```python
from build123d import *

# Parameters (mm, degrees)
SKETCH_1_R          = 14
SKETCH_1_R_2        = 1.5
EXTRUDE_1_DEPTH     = 2
CUT_EXTRUDE_1_DEPTH = 20.899748742
EXTRUDE_4_DEPTH     = 1
SKETCH_6_R          = 7
SKETCH_6_R_2        = 3.1
EXTRUDE_5_DEPTH     = 5
EXTRUDE_6_DEPTH     = 1
SKETCH_8_W          = 8
SKETCH_8_H          = 2
EXTRUDE_7_DEPTH     = 5
SKETCH_9_R          = 1.6
CUT_EXTRUDE_3_DEPTH = 24.108440017
EXTRUDE_8_DEPTH     = 2
SKETCH_11_W         = 12.041493288
SKETCH_11_H         = 2
CUT_EXTRUDE_4_DEPTH = 5
SKETCH_12_R         = 20
SKETCH_12_R_2       = 3.1
EXTRUDE_9_DEPTH     = 2
SKETCH_13_R         = 2.3
CUT_EXTRUDE_5_DEPTH = 2
CUT_EXTRUDE_START   = -1
CUT_EXTRUDE_6_DEPTH = 1
FILLET_1_R          = 3
FILLET_2_R          = 1.5
SKETCH_15_R         = 20
CUT_EXTRUDE_7_DEPTH = 2
SKETCH_16_R         = 7
CUT_EXTRUDE_8_DEPTH = 5


with BuildPart() as part:
    # 草图1 → 凸台-拉伸1 (new body)
    with BuildSketch(Plane.XY):
        Circle(SKETCH_1_R)
        with Locations((-7.071067812, 7.071067812)):
            Circle(SKETCH_1_R_2, mode=Mode.SUBTRACT)
        with Locations((7.071067812, 7.071067812)):
            Circle(SKETCH_1_R_2, mode=Mode.SUBTRACT)
        with Locations((-7.071067812, -7.071067812)):
            Circle(SKETCH_1_R_2, mode=Mode.SUBTRACT)
        with Locations((7.071067812, -7.071067812)):
            Circle(SKETCH_1_R_2, mode=Mode.SUBTRACT)
    extrude(amount=EXTRUDE_1_DEPTH)

    # 草图2 → 切除-拉伸1 (cut, through all)
    with BuildSketch(Plane(origin=(0, 0, 0), x_dir=(-1, 0, 0), z_dir=(0, 0, -1))):
        with BuildLine():
            ThreePointArc((-2.683281573, 3.1), (-4.1, 0), (-2.683281573, -3.1))
            Line((-2.683281573, -3.1), (2.683281573, -3.1))
            ThreePointArc((2.683281573, -3.1), (4.1, 0), (2.683281573, 3.1))
            Line((2.683281573, 3.1), (-2.683281573, 3.1))
        make_face()
    extrude(amount=-CUT_EXTRUDE_1_DEPTH, mode=Mode.SUBTRACT)

    # 草图3 → 凸台-拉伸4 (add)
    with BuildSketch(Plane(origin=(0, 0, 0), x_dir=(-1, 0, 0), z_dir=(0, 0, -1))):
        Polygon((0, 3.1), (3.7, 3.1), (3.7, 7.1), (-3.7, 7.1), (-3.7, 3.1), align=None)
    extrude(amount=EXTRUDE_4_DEPTH)

    # 草图6 → 凸台-拉伸5 (add)
    with BuildSketch(Plane(origin=(0, 0, -1), x_dir=(-1, 0, 0), z_dir=(0, 0, -1))):
        with Locations(Location((0, 0, 0), (0, 0, 121.908982735))):
            Circle(SKETCH_6_R)
        with Locations(Location((0, 0, 0), (0, 0, 90))):
            Circle(SKETCH_6_R_2, mode=Mode.SUBTRACT)
    extrude(amount=EXTRUDE_5_DEPTH)

    # 草图7 → 凸台-拉伸6 (add)
    with BuildSketch(Plane(origin=(0, 0, -6), x_dir=(-1, 0, 0), z_dir=(0, 0, -1))):
        with BuildLine():
            Line((-2.5, 3.1), (-2.5, 6.538348415))
            ThreePointArc((-2.5, 6.538348415), (0, 7), (2.5, 6.538348415))
            Line((2.5, 6.538348415), (2.5, 3.1))
            Line((2.5, 3.1), (-2.5, 3.1))
        make_face()
    extrude(amount=EXTRUDE_6_DEPTH)

    # 草图8 → 凸台-拉伸7 (add)
    with BuildSketch(Plane(origin=(0, 0, -6), x_dir=(-1, 0, 0), z_dir=(0, 0, -1))):
        with Locations((9.447401339, 2)):
            Rectangle(SKETCH_8_W, SKETCH_8_H)
        with Locations((9.447401339, -2)):
            Rectangle(SKETCH_8_W, SKETCH_8_H)
    extrude(amount=-EXTRUDE_7_DEPTH)

    # 草图9 → 切除-拉伸3 (cut, through all)
    with BuildSketch(Plane(origin=(0, 3, 0), x_dir=(1, 0, 0), z_dir=(0, 1, 0))):
        with Locations(Location((-10.8, 4, 0), (0, 0, 180))):
            Circle(SKETCH_9_R)
    extrude(amount=-CUT_EXTRUDE_3_DEPTH, mode=Mode.SUBTRACT)

    # 草图10 → 凸台-拉伸8 (add)
    with BuildSketch(Plane(origin=(0, 0, -7), x_dir=(-1, 0, 0), z_dir=(0, 0, -1))):
        with BuildLine():
            Line((-2.5, 6.538348415), (-2.5, 3.1))
            ThreePointArc((-2.5, 3.1), (0, -3.98246155), (2.5, 3.1))
            Line((2.5, 3.1), (2.5, 6.538348415))
            ThreePointArc((2.5, 6.538348415), (0, 7), (-2.5, 6.538348415))
        make_face()
    extrude(amount=EXTRUDE_8_DEPTH)

    # 草图11 → 切除-拉伸4 (cut)
    with BuildSketch(Plane(origin=(0, 0, -6), x_dir=(-1, 0, 0), z_dir=(0, 0, -1))):
        with Locations((7.426654695, 0)):
            Rectangle(SKETCH_11_W, SKETCH_11_H)
    extrude(amount=-CUT_EXTRUDE_4_DEPTH, mode=Mode.SUBTRACT)

    # 草图12 → 凸台-拉伸9 (add)
    with BuildSketch(Plane.XY.offset(2)):
        Circle(SKETCH_12_R)
        Circle(SKETCH_12_R_2, mode=Mode.SUBTRACT)
    extrude(amount=-EXTRUDE_9_DEPTH)

    # 草图13 → 切除-拉伸5 (cut)
    with BuildSketch(Plane.XY.offset(2)):
        with Locations((10.253048327, 10.253048327)):
            Circle(SKETCH_13_R)
        with Locations((-10.253048327, 10.253048327)):
            Circle(SKETCH_13_R)
        with Locations((-10.253048327, -10.253048327)):
            Circle(SKETCH_13_R)
        with Locations((10.253048327, -10.253048327)):
            Circle(SKETCH_13_R)
    extrude(amount=-CUT_EXTRUDE_5_DEPTH, mode=Mode.SUBTRACT)

    # 草图14 → 切除-拉伸6 (cut)
    with BuildSketch(Plane(origin=(0, 0, -1), x_dir=(-1, 0, 0), z_dir=(0, 0, -1)).offset(CUT_EXTRUDE_START)):
        with BuildLine():
            Line((-4.590882623, 5.284297185), (-4.590882623, 9.738638689))
            Line((-4.590882623, 9.738638689), (4.724825977, 9.738638689))
            Line((4.724825977, 9.738638689), (4.724825977, 5.164883298))
            ThreePointArc((4.724825977, 5.164883298), (0.089722487, 6.999424967), (-4.590882623, 5.284297185))
        make_face()
    extrude(amount=CUT_EXTRUDE_6_DEPTH, mode=Mode.SUBTRACT)

    # 圆角1
    fillet_1_edges = [part.edges().sort_by_distance(p)[0] for p in [
        (0, 7, -9),
    ]]
    fillet(fillet_1_edges, radius=FILLET_1_R)

    # 圆角2
    fillet_2_edges = [part.edges().sort_by_distance(p)[0] for p in [
        (-13.447401339, -2, -1),
        (-13.447401339, -2, -6),
        (-13.447401339, 2, -1),
        (-13.447401339, 2, -6),
    ]]
    fillet(fillet_2_edges, radius=FILLET_2_R)

    # 草图15 → 切除-拉伸7 (cut)
    with BuildSketch(Plane.XY.offset(2)):
        Circle(SKETCH_15_R)
    extrude(amount=-CUT_EXTRUDE_7_DEPTH, mode=Mode.SUBTRACT)

    # 草图16 → 切除-拉伸8 (cut)
    with BuildSketch(Plane(origin=(0, 0, -6), x_dir=(-1, 0, 0), z_dir=(0, 0, -1))):
        Circle(SKETCH_16_R)
    extrude(amount=CUT_EXTRUDE_8_DEPTH, mode=Mode.SUBTRACT)


solid = part.part
```
Here's how the part is built. I have some questions about the finished solid (model axes, mm). A direction names the side the tool comes from. Round coordinates to 2 decimals unless told otherwise and drop trailing zeros. Order: outer loops, then holes, each group sorted by start corner. A loop starts at its lowest first (then second) coordinate and runs counter-clockwise, first axis right, second up. Notation, with made-up numbers: M 17,49 L 21,49 A15 ccw 21,53 Z; hole C -8.5,69 d4. An arc over 180 degrees is marked long. Answer in a Markdown table with one row per item.
Item 1: Imagine slicing it at B-B, the plane x = -10.8. Write out the boundary of the cut face in (y, z), and give its area (3 significant figures).
A:
| item | result |
|---|---|
| outline | M -3,-6 L -1,-6 L -1,-5.6 L -3,-5.6 Z; M -3,-2.4 L -1,-2.4 L -1,-1 L -3,-1 Z; M 1,-6 L 3,-6 L 3,-5.6 L 1,-5.6 Z; M 1,-2.4 L 3,-2.4 L 3,-1 L 1,-1 Z |
| area | 7.20 mm2 |
Item 2: For faces 4 (the face through (-9, 3, -4)), 5 (the face through (0.1, 3.1, -0.5)), 6 (the face through (-3.7, 4.5, -0.5)), which set-ups out of +Z, -Z, +X, -X, +Y, -Y let a thin tool reach every point of the face, with its end or its side?
A:
| item | result |
|---|---|
| face 4 | +Z, -Z, -X, +Y |
| face 5 | +Z, +X, -X, -Y |
| face 6 | +Z, -X, +Y, -Y |
Item 3: If I drill on L1, parallel to Y at x = -10.25, z = -5.65; L2, parallel to Y at x = -5, z = -3.2; L3, parallel to Z at x = -5.75, y = 2, over which ranges is the centre line in solid material (lowest first)? Write a range as from..to.
A:
| item | result |
|---|---|
| L1 | y = -3..-1, 1..3 |
| L2 | y = -4.9..-1, 1..4.9 |
| L3 | z = -6..-1 |
Item 4: I'm going to push flat-ended pins straight in: pin 1 (2.5 mm diameter, centred on x = -10.5, z = -4.5, fed in from -Y); pin 2 (3 mm diameter, centred on x = -4, z = -4.5, fed in from -Y); pin 3 (1.5 mm diameter, centred on y = -4.5, z = -1.5, fed in from +X). Where does each tip first touch, or does it pass through?
A:
| item | result |
|---|---|
| pin 1 | stops at y = -3 |
| pin 2 | stops at y = -6.54 |
| pin 3 | stops at x = 5.91 |
Item 5: Imagine slicing it at A-A, the plane z = -4. Write out the boundary of the cut face in (x, y), and give its area (3 significant figures).
A:
| item | result |
|---|---|
| outline | M -13.45,-3 L -12.4,-3 L -12.4,-1 L -13.45,-1 Z; M -13.45,1 L -12.4,1 L -12.4,3 L -13.45,3 Z; M -9.2,-3 L -6.32,-3 A7 ccw long -6.32,3 L -9.2,3 L -9.2,1 L -2.93,1 A3.1 cw long -2.93,-1 L -9.2,-1 Z |
| area | 130 mm2 |
Item 6: Imagine slicing it at D-D, the plane x = -8. Write out the boundary of the cut face in (y, z), and give its area (3 significant figures).
A:
| item | result |
|---|---|
| outline | M -3,-6 L -1,-6 L -1,-1 L -3,-1 Z; M 1,-6 L 3,-6 L 3,-1 L 1,-1 Z |
| area | 20.0 mm2 |
Item 7: Thinking about a two-plate mould opening in Y: for faces 1 (the face through (3.7, 4.5, -0.5)), 2 (the face through (-9, -3, -4)), 3 (the face through (-8, 1, -4)), which applies, +Y half, -Y half, draft (parallel to the pull), parting line (faces both ways), or undercut?
A:
| item | result |
|---|---|
| face 1 | draft |
| face 2 | -Y half |
| face 3 | undercut |
Item 8: Imagine slicing it at C-C, the plane y = -1.75. Write out the boundary of the cut face in (x, z).
A:
| item | result |
|---|---|
| outline | M -13.45,-4.5 A1.5 ccw -11.95,-6 L -2.56,-6 L -2.56,-1 L -11.95,-1 A1.5 ccw -13.45,-2.5 Z; M 2.56,-6 L 6.78,-6 L 6.78,-1 L 2.56,-1 Z; hole C -10.8,-4 d3.2 |
